Autodesk Inventor part; units mm, degrees
ref_plane "YZ Plane" through (0, 0, 0) normal (1, 0, 0) x (0, 1, 0)
ref_plane "XZ Plane" through (0, 0, 0) normal (0, 1, 0) x (-1, 0, 0)
ref_plane "XY Plane" through (0, 0, 0) normal (0, 0, 1) x (1, 0, 0)
sketch "Sketch1" plane through (0, 0, 0) normal (0, 0, 1) x (1, 0, 0)
  line L0 (0, 0) -> (24.13, 0)
  line L1 (24.13, 0) -> (24.13, -32.385)
  line L2 (24.13, -32.385) -> (0, -32.385)
  line L3 (0, -32.385) -> (0, 0)
  dimension "d0" = 24.13
  dimension "d1" = 32.385
extrude "Extrusion1" add sketch "Sketch1" along normal blind 27.94
sketch "Sketch2" plane through (24.13, -32.385, 0) normal (1, 0, 0) x (0, 0, -1)
  line L0 (-27.94, 29.083) -> (-3.302, 29.083)
  line L1 (-3.302, 29.083) -> (-3.302, 3.302)
  line L2 (-3.302, 3.302) -> (-27.94, 3.302)
  line L3 (-27.94, 3.302) -> (-27.94, 29.083)
  line L4 (-27.94, 0) -> (-27.94, 32.385)
  line L5 (0, 0) -> (-27.94, 0)
  line L6 (0, 32.385) -> (0, 0)
  line L7 (0, 32.385) -> (-27.94, 32.385)
  dimension "d4" = 0
  dimension "d5" = 3.302
  dimension "d6" = 3.302
  dimension "d7" = 3.302
extrude "Extrusion2" cut sketch "Sketch2" against normal blind 34.925 contours L0 L1 L2 L3
sketch "Sketch3" plane through (24.13, -29.083, 3.302) normal (0, 0, 1) x (1, 0, 0)
  line L0 (-24.13, 0) -> (-24.13, 25.781)
  line L1 (0, 0) -> (-24.13, 0)
  line L2 (0, 25.781) -> (0, 0)
  line L3 (0, 25.781) -> (-24.13, 25.781)
  line L4 (-24.13, 25.781) -> (0, 25.781)
  line L5 (-12.065, 25.781) -> (-12.065, 0)
  line L6 (0, 0) -> (-24.13, 0)
  line L7 (-24.13, 0) -> (-24.13, 25.781)
  line L8 (-24.13, 12.8905) -> (0, 12.8905)
  circle A0 centre (-12.065, 12.8905) radius 3.175
  point P0 (-24.13, 29.083)
  dimension "d10" = 6.35
extrude "Extrusion3" cut sketch "Sketch3" against normal blind 34.925 contours A0 L5 L8 | L8 L5 A0 | L5 L8 A0 | L5 A0 L8
fillet "Fillet1" radius 3.175 2 edges at (12.065, 0, 0) (12.065, -32.385, 0)
sketch "Sketch4" plane through (0, 0, 27.94) normal (0, 1, 0) x (1, 0, 0)
  circle A0 centre (12.065, 12.319) radius 3.175
  line L0 (24.13, 24.765) -> (24.13, 0)
  line L1 (24.13, 0) -> (0, 0)
  point P0 (0, 27.94)
  dimension "d14" = 6.35
  dimension "d15" = 12.065
  dimension "d16" = 12.319
extrude "Extrusion4" cut sketch "Sketch4" against normal blind 34.925
properties part number "RobotArm CylinderPart2"
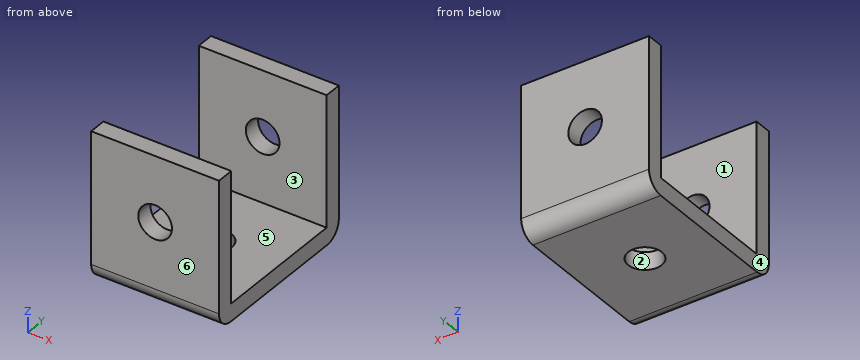
Build history of the part. All positions in model axes, mm. Face numbers are marked on the shaded views. A direction names the side the tool comes from. Give positions to 0.01 mm unless a question says otherwise; leave off trailing zeros. Order: outer loops, then holes, each group sorted by start corner. A loop starts at its lowest first (then second) coordinate and runs counter-clockwise, first axis right, second up. Notation, with made-up numbers: M 0.25,-39.75 L 17.25,-39.75 A20 ccw 17.25,-22.75 Z; hole C 67.5,67.5 d11. An arc over 180 degrees is marked long. Put each result on its own line as item: value.
Item 1: Which spindle directions (+Z, -Z, +X, -X, +Y, -Y) get a long thin tool onto all of the face, cutting with end or side? Do the marked faces 1 and 2. Say none if no direction does.
Results are:
face 1: +Z, +X, -X
face 2: +Z, -Z
Item 2: Cut at D-D on y = -4. Write the cut outline in (x, z).
Results are:
outline: M 0,0 L 24.13,0 L 24.13,3.3 L 0,3.3 Z
Item 3: Drop flat-ended pins along their axis: pin 1 Ø6 at (x, y) = (14, -5.5) entering from -Z; pin 2 Ø4 at (x, z) = (12.065, 15.621) entering from -Y. Give the stop position or say it passes through.
Results are:
pin 1: z = 0
pin 2: through
Item 4: Pull direction Y, two halves, no side cores. Call the marked faces 3, 4, 5 and 6: +Y half, -Y half, draft (parallel to the pull), parting line (faces both ways), or undercut.
Results are:
face 3: undercut
face 4: draft
face 5: undercut
face 6: -Y half
Item 5: Cut at C-C on z = 13.5. Write the cut outline in (x, y) (3 decimals).
Results are:
outline: M 0,-32.385 L 9.702,-32.385 L 9.702,-29.083 L 0,-29.083 Z; M 0,-3.302 L 9.702,-3.302 L 9.702,0 L 0,0 Z; M 14.428,-32.385 L 24.13,-32.385 L 24.13,-29.083 L 14.428,-29.083 Z; M 14.428,-3.302 L 24.13,-3.302 L 24.13,0 L 14.428,0 Z
Item 6: Cut at B-B on x = 6. Write the cut outline in (y, z) (3 decimals).
Results are:
outline: M -32.385,3.175 A3.175 ccw -29.21,0 L -3.175,0 A3.175 ccw 0,3.175 L 0,27.94 L -3.302,27.94 L -3.302,3.302 L -29.083,3.302 L -29.083,27.94 L -32.385,27.94 Z
Item 7: Cut at A-A on z = 22.25. Write the cut outline in (x, y) (3 decimals).
Results are:
outline: M 0,-32.385 L 24.13,-32.385 L 24.13,-29.083 L 0,-29.083 Z; M 0,-3.302 L 24.13,-3.302 L 24.13,0 L 0,0 Z
Item 8: Wall check: probe 1 along Y at (x, z) = (13.25, 4.5) (3 decimals); probe 2 along Z at (x, y) = (3.5, -10.5); probe 3 along Z at (x, y) = (3, -3). Give the ranges that are in metal, low to high.
Results are:
probe 1: -32.385 to -29.083, -3.302 to 0
probe 2: 0 to 3.3
probe 3: 0 to 27.94
